Can you work these out from the model? Positions are in its coordinate system, mm. Face numbers are marked on the shaded views. A direction names the side the tool comes from. Coordinates: 2 decimals unless noted, no trailing zeros. Order: outer loops, then holes, each group sorted by start corner. A loop starts at its lowest first (then second) coordinate and runs counter-clockwise, first axis right, second up. Notation, with made-up numbers: (75.5, 38) - (107.5, 38) arc R38 ccw to (107.5, 77) - close; hole circle Ø4 at (29, -22.5). An arc over 180 degrees is marked (long way). Use a Markdown table: item, result. Add a question column.
(1) On a 3-axis mill with a long thin cutter (end or side, diameter ignored), from which of +Z, -Z, +X, -X, +Y, -Y can I reach the whole of each face in a straight line? I mean the marked faces 4, 5, 6 and 7. Say none if no direction works.
(2) We'd pull the mould along Y, two halves only. Please class the marked faces 1, 2 and 3: pulls with the +Y half, pulls with the -Y half, needs draft (parallel to the pull), parting line crosses it, or undercut.
(3) I want a section at A-A (x = 71). List the corners of the cut face in (y, z) for me, and give its area (3 significant figures).
(4) For pin 1 Ø5.5 at (x, y) = (0.5, -8) entering from -Z; pin 2 Ø4 at (y, z) = (46.99, 9.525) entering from +X; pin 3 Ø8 at (y, z) = (-9, 11.5) entering from +X; pin 4 Ø3.5 at (y, z) = (46.99, 9.525) entering from +X, each with a flat end and sliding along its axis, tell me the tip position at first contact or that it passes through.
(5) If I drill on L1, parallel to Y at x = 55.5, z = 10.75; L2, parallel to Z at x = -5.2, y = -11.43 (3 decimals); L3, parallel to X at y = 1.5, z = 16, over which ranges is the centre line in solid material (lowest first)? Write a range as [from, to].
(6) I want a section at B-B (z = 16.25). State how many separate pieces and enclosed holes the cut face has, and give its area (3 significant figures).
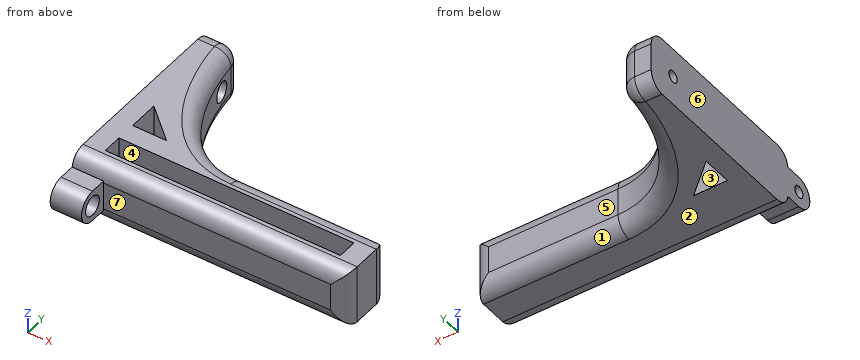
```python
from build123d import *

# Parameters (mm, degrees)
F0_W      = 76.2
F0_H      = 6.35
F1_DEPTH  = 19.05
F2_DEPTH  = 6.35
F4_START  = -5.08
F3_R      = 3.175
F3_R_2    = 1.905
F4_DEPTH  = 6.8182960521
F6_DEPTH  = 10.16
F7_R      = 3.175
F7_R_2    = 1.905
F8_DEPTH  = 5.08
F9_DEPTH  = 10.1610001
F10_DEPTH = 88.9010001
F11_R     = 5.08


with BuildPart() as f1:
    # F0 (on Top) → F1 (new body)
    with BuildSketch(Plane.XY):
        with BuildLine():
            Line((-6.35, -6.35), (82.55, -6.35))
            Line((82.55, -6.35), (82.55, 12.7))
            Line((82.55, 12.7), (35.4121256149, 12.7))
            add(Edge.make_bspline(
                [(3.81, 57.15), (3.81, 44.45), (10.9720126255, 12.7), (35.4121256149, 12.7)],
                knots=[0, 0, 0, 0, 54.538947949, 54.538947949, 54.538947949, 54.538947949], degree=3))
            Line((3.81, 57.15), (-6.35, 57.15))
            Line((-6.35, 57.15), (-6.35, 12.7))
            Line((-6.35, 12.7), (-6.35, -6.35))
        make_face()
        Polygon((0, 12.7), (0, 22.5350875407), (10.9720126255, 12.7), align=None, mode=Mode.SUBTRACT)
        with Locations((38.1, 3.175)):
            Rectangle(F0_W, F0_H, mode=Mode.SUBTRACT)
    extrude(amount=F1_DEPTH)

    # F0 (on Top) → F2 (join)
    with BuildSketch(Plane.XY):
        with Locations((38.1, 3.175)):
            Rectangle(F0_W, F0_H)
    extrude(amount=F2_DEPTH)

    # F3 (on face) → F4 (cut)
    with BuildSketch(Plane(origin=(-6.35, 0, 0), x_dir=(0, -1, 0), z_dir=(-1, 0, 0)).offset(F4_START)):
        with Locations((-46.99, 9.525)):
            Circle(F3_R)
        with Locations((-46.99, 9.525)):
            Circle(F3_R_2, mode=Mode.SUBTRACT)
    extrude(amount=-F4_DEPTH, mode=Mode.SUBTRACT)

    # F5 (on face) → F6 (join)
    with BuildSketch(Plane(origin=(-6.35, 0, 0), x_dir=(0, -1, 0), z_dir=(-1, 0, 0))):
        with BuildLine():
            Line((11.43, 14.605), (6.35, 14.605))
            Line((6.35, 14.605), (6.35, 4.445))
            Line((6.35, 4.445), (11.43, 4.445))
            ThreePointArc((11.43, 4.445), (16.51, 9.525), (11.43, 14.605))
        make_face()
    extrude(amount=-F6_DEPTH)

    # F7 (on face) → F8 (cut)
    with BuildSketch(Plane.YZ.offset(3.81)):
        with Locations((-11.43, 9.525)):
            Circle(F7_R)
        with Locations((-11.43, 9.525)):
            Circle(F7_R_2, mode=Mode.SUBTRACT)
    extrude(amount=-F8_DEPTH, mode=Mode.SUBTRACT)

    # F7 (on face) → F9 (cut, through all)
    with BuildSketch(Plane.YZ.offset(3.81)):
        with Locations((-11.43, 9.525)):
            Circle(F7_R_2)
    extrude(amount=-F9_DEPTH, mode=Mode.SUBTRACT)

    # F3 (on face) → F10 (cut, through all)
    with BuildSketch(Plane(origin=(-6.35, 0, 0), x_dir=(0, -1, 0), z_dir=(-1, 0, 0))):
        with Locations((-46.99, 9.525)):
            Circle(F3_R_2)
    extrude(amount=-F10_DEPTH, mode=Mode.SUBTRACT)

    # F11
    f11_edges = [f1.edges().sort_by_distance(p)[0] for p in [
        (58.981063, 12.7, 0),
        (58.981063, 12.7, 19.05),
        (38.1, -6.35, 19.05),
        (38.1, -6.35, 0),
        (82.55, -6.35, 9.525),
        (82.55, 12.7, 9.525),
        (3.81, 57.15, 9.525),
        (-1.27, 57.15, 19.05),
        (-1.27, 57.15, 0),
    ]]
    fillet(f11_edges, radius=F11_R)


solid = f1.part
```
Answers follow:
| question | item | result |
|---|---|---|
| 1 | face 4 | +Z |
| 1 | face 5 | +Z, -Z, +X, +Y |
| 1 | face 6 | +Z, -Z, -X, +Y, -Y |
| 1 | face 7 | +Z, -Z, +X, -Y |
| 2 | face 1 | pulls with the +Y half |
| 2 | face 2 | needs draft |
| 2 | face 3 | undercut |
| 3 | outline | (-6.35, 5.08) arc R5.08 ccw to (-1.27, 0) - (7.62, 0) arc R5.08 ccw to (12.7, 5.08) - (12.7, 13.97) arc R5.08 ccw to (7.62, 19.05) - (6.35, 19.05) - (6.35, 6.35) - (0, 6.35) - (0, 19.05) - (-1.27, 19.05) arc R5.08 ccw to (-6.35, 13.97) - close |
| 3 | area | 260 mm² |
| 4 | pin 1 | stops at z = 1.92 |
| 4 | pin 2 | stops at x = -1.27 |
| 4 | pin 3 | stops at x = 80.92 |
| 4 | pin 4 | passes through |
| 5 | L1 | y = [-6.35, 0], [6.35, 12.7] |
| 5 | L2 | z = [4.445, 7.62], [11.43, 14.605] |
| 5 | L3 | x = [-6.35, 0], [76.2, 82.55] |
| 6 | separate pieces | 1 |
| 6 | enclosed holes | 2 |
| 6 | area | 1,790 mm² |
